from build123d import *

# Parameters (mm, degrees)
PAD002_DEPTH          = 10.75
SKETCH034_W           = 20.5
SKETCH034_H           = 9
SKETCH034_W_2         = 10
SKETCH034_H_2         = 18
POCKET004_DEPTH       = 5
SKETCH035_R           = 0.25
POCKET005_DEPTH       = 9.25
CLONE_PLACEMENT_ANGLE = 180


with BuildPart() as part:
    # Sketch033 → Pad002 (new body, symmetric)
    with BuildSketch(Plane.YZ):
        with BuildLine():
            Line((21.8202830187, 8.7154073795), (26.7049742837, 7.6477973171))
            ThreePointArc((26.0644082463, 4.7169825581), (27.8500986445, 5.8621069189), (26.7049742837, 7.6477973171))
            Line((26.0644082463, 4.7169825581), (21.1797169813, 5.7845926205))
            ThreePointArc((21.8202830187, 8.7154073795), (20.0345926205, 7.5702830187), (21.1797169813, 5.7845926205))
        make_face()
    extrude(amount=PAD002_DEPTH, both=True)

    # Sketch034 (on Face3 of Pad002) → Pocket004 (cut)
    with BuildSketch(Plane(origin=(0, 2.812837698, 12.869721088), x_dir=(0, -0.976938253, 0.2135220125), z_dir=(0, 0.2135220125, 0.976938253))):
        with Locations((-10.25, 0)):
            Rectangle(SKETCH034_W, SKETCH034_H)
        with Locations((-27.25, 0)):
            Rectangle(SKETCH034_W_2, SKETCH034_H_2)
    extrude(amount=-POCKET004_DEPTH, mode=Mode.SUBTRACT)

    # Sketch035 → Pocket005 (cut, symmetric)
    with BuildSketch(Plane.YZ):
        with Locations((26.384691265, 6.1823899376)):
            Circle(SKETCH035_R)
    extrude(amount=POCKET005_DEPTH, both=True, mode=Mode.SUBTRACT)


with BuildPart() as part_1:
    # Clone placement: moved
    add(part.part.rotate(Axis((0, 0, 0), (0, 0, 1)), CLONE_PLACEMENT_ANGLE))


solid = part_1.part
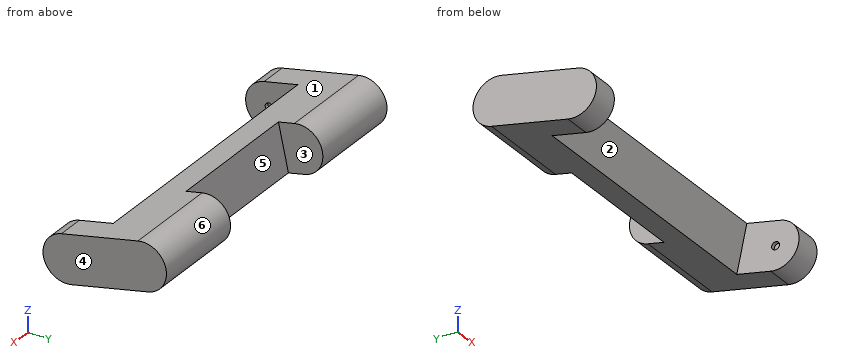
Could you check a few things on this model? Use its own coordinates, in mm. Face numbers are marked on the shaded views. A direction names the side the tool comes from. Round coordinates to 2 decimals unless told otherwise and drop trailing zeros. Write each loop counter-clockwise with the first axis right and the second up, starting at its lowest first coordinate (ties: lowest second). Pieces come first, ordered by that corner, then holes. Notation, with made-up numbers: (60, 44) - (114, 44) arc R16 cw to (114, 50) - close; hole circle Ø8 at (20.5, -27). An arc over 180 degrees is marked (long way). Use a Markdown table: item, result.
Q1. For pin 1 (1.5 mm diameter, centred on x = -3, z = 6.5, fed in from +Y); pin 2 (3 mm diameter, centred on x = 3, y = -22.5, fed in from -Z), each with a flat end and sliding along its axis, tell me the tip position at first contact or that it passes through.
Output values:
| item | result |
|---|---|
| pin 1 | y = -22.24 |
| pin 2 | z = 5.19 |
Q2. I want a section at D-D (y = -27). List the corners of the cut face in (x, z) for me.
Output values:
| item | result |
|---|---|
| outline | (-10.75, 4.81) - (-9, 4.81) - (-9, 7.55) - (-10.75, 7.55) - close; (9, 4.81) - (10.75, 4.81) - (10.75, 7.55) - (9, 7.55) - close |
Q3. I want a section at A-A (y = -20.5). List the corners of the cut face in (x, z) for me.
Output values:
| item | result |
|---|---|
| outline | (-10.75, 6.13) - (-4.5, 6.13) - (-4.5, 8.37) - (-10.75, 8.37) - close; (4.5, 6.13) - (10.75, 6.13) - (10.75, 8.37) - (4.5, 8.37) - close |
Q4. I want a section at B-B (z = 7.4). List the corners of the cut face in (x, y) for me.
Output values:
| item | result |
|---|---|
| outline | (-10.75, -27.26) - (-9, -27.26) - (-9, -24.39) - (9, -24.39) - (9, -27.26) - (10.75, -27.26) - (10.75, -20.01) - (4.5, -20.01) - (4.5, -22.6) - (-4.5, -22.6) - (-4.5, -20.01) - (-10.75, -20.01) - close |
Q5. Please list where these lines run through material, in increasing order: L1, parallel to X at y = -26, z = 5.8; L2, parallel to X at y = -21.75, z = 7.05; L3, parallel to Z at x = -10, y = -22.25.
Output values:
| item | result |
|---|---|
| L1 | -10.75 to -9, 9 to 10.75 |
| L2 | -10.75 to -4.5, 4.5 to 10.75 |
| L3 | 5.55 to 8.62 |
Q6. For the marked faces 1 and 2, which set-ups out of +Z, -Z, +X, -X, +Y, -Y let a thin tool reach every point of the face, with its end or its side?
Output values:
| item | result |
|---|---|
| face 1 | +Z, +X, -X, -Y |
| face 2 | -Z, -Y |
Q7. I want a section at C-C (x = 3). List the corners of the cut face in (y, z) for me.
Output values:
| item | result |
|---|---|
| outline | (-24.55, 8.12) - (-23.91, 5.19) - (-22.2, 5.56) - (-22.84, 8.49) - close |
Q8. Thinking about a two-plate mould opening in X: for the marked faces 3, 4, 5 and 6, which applies, released by +X, released by -X, zero draft, split by the parting line, or undercut?
Output values:
| item | result |
|---|---|
| face 3 | undercut |
| face 4 | released by +X |
| face 5 | undercut |
| face 6 | zero draft |
